from build123d import *

# Parameters (mm, degrees)
F0_R     = 13.5
F0_R_2   = 2.4852724595
F1_DEPTH = 7


with BuildPart() as f1:
    # F0 (on Top) → F1 (new body)
    with BuildSketch(Plane.XY):
        Circle(F0_R)
        with BuildLine():
            ThreePointArc((-11.0212433186, 4.5651484568), (-9.9188569362, 6.6275683173), (-8.4352944442, 8.4352944442))
            ThreePointArc((-8.4352944442, 8.4352944442), (-6.6275683173, 9.9188569362), (-4.5651484568, 11.0212433186))
            ThreePointArc((-4.5651484568, 11.0212433186), (-2.3272925012, 11.7000895011), (0, 11.9293078056))
            ThreePointArc((0, 11.9293078056), (2.3272925012, 11.7000895011), (4.5651484568, 11.0212433186))
            ThreePointArc((4.5651484568, 11.0212433186), (6.6275683173, 9.9188569362), (8.4352944442, 8.4352944442))
            ThreePointArc((8.4352944442, 8.4352944442), (9.9188569362, 6.6275683173), (11.0212433186, 4.5651484568))
            ThreePointArc((11.0212433186, 4.5651484568), (11.7000895011, 2.3272925012), (11.9293078056, 0))
            ThreePointArc((11.9293078056, 0), (11.7000895011, -2.3272925012), (11.0212433186, -4.5651484568))
            ThreePointArc((11.0212433186, -4.5651484568), (9.9188569362, -6.6275683173), (8.4352944442, -8.4352944442))
            ThreePointArc((8.4352944442, -8.4352944442), (6.6275683173, -9.9188569362), (4.5651484568, -11.0212433186))
            ThreePointArc((4.5651484568, -11.0212433186), (2.3272925012, -11.7000895011), (0, -11.9293078056))
            ThreePointArc((0, -11.9293078056), (-2.3272925012, -11.7000895011), (-4.5651484568, -11.0212433186))
            ThreePointArc((-4.5651484568, -11.0212433186), (-6.6275683173, -9.9188569362), (-8.4352944442, -8.4352944442))
            ThreePointArc((-8.4352944442, -8.4352944442), (-9.9188569362, -6.6275683173), (-11.0212433186, -4.5651484568))
            ThreePointArc((-11.0212433186, -4.5651484568), (-11.7000895011, -2.3272925012), (-11.9293078056, 0))
            ThreePointArc((-11.9293078056, 0), (-11.7000895011, 2.3272925012), (-11.0212433186, 4.5651484568))
        make_face(mode=Mode.SUBTRACT)
        with BuildLine():
            add(Edge.make_bspline(
                [(11.0212433186, 4.5651484568), (10.7307703614, 1.5514252721), (10.1663660438, -4.1433714543), (2.2942810987, -7.8104935299), (-0.1989491839, -4.6915291397), (-1.3315016332, -3.2145293013)],
                knots=[0, 0, 0, 0, 0.3754408897, 0.7085801344, 1, 1, 1, 1], degree=3))
            ThreePointArc((-1.3315016332, -3.2145293013), (-1.9330407592, -2.8929999397), (-2.4602942129, -2.4602942129))
            add(Edge.make_bspline(
                [(11.9293078056, 0), (10.5030009531, -2.6730846833), (7.8115947966, -7.7171301221), (-0.8744432081, -8.0954908894), (-1.9556350248, -4.2535609012), (-2.4602942129, -2.4602942129)],
                knots=[0, 0, 0, 0, 0.3754632807, 0.7084900303, 1, 1, 1, 1], degree=3))
            ThreePointArc((11.9293078056, 0), (11.7000895011, 2.3272925012), (11.0212433186, 4.5651484568))
        make_face()
        with BuildLine():
            add(Edge.make_bspline(
                [(4.5651484568, 11.0212433186), (6.4882912926, 8.6805285734), (10.1197801342, 4.2634610727), (7.1432551055, -3.9049968446), (3.1838363189, -3.436219375), (1.3315016332, -3.2145293013)],
                knots=[0, 0, 0, 0, 0.3754632807, 0.7084900303, 1, 1, 1, 1], degree=3))
            ThreePointArc((1.3315016332, -3.2145293013), (0.6787936462, -3.4125261045), (0, -3.4793814433))
            add(Edge.make_bspline(
                [(8.4352944442, 8.4352944442), (9.3162939954, 5.5368010983), (10.9810136566, 0.0662522262), (5.1051295916, -6.3413520413), (1.6264969852, -4.3930541604), (0, -3.4793814433)],
                knots=[0, 0, 0, 0, 0.3754632807, 0.7084900303, 1, 1, 1, 1], degree=3))
            ThreePointArc((8.4352944442, 8.4352944442), (6.6275683173, 9.9188569362), (4.5651484568, 11.0212433186))
        make_face()
        with BuildLine():
            add(Edge.make_bspline(
                [(-4.5651484568, 11.0212433186), (-1.5653669998, 10.7472190798), (4.1505997502, 10.2265263001), (7.9846135159, 1.9883168119), (4.7170514854, -0.2873495043), (3.2145293013, -1.3315016332)],
                knots=[0, 0, 0, 0, 0.3743391134, 0.7130961412, 1, 1, 1, 1], degree=3))
            ThreePointArc((3.2145293013, -1.3315016332), (2.8692477592, -1.968124113), (2.399653463, -2.5194758355))
            add(Edge.make_bspline(
                [(0, 11.9293078056), (2.6660813096, 10.5051188653), (7.7130575447, 7.806165889), (8.1160713079, -0.8810343308), (4.1864871277, -1.9887456195), (2.399653463, -2.5194758355)],
                knots=[0, 0, 0, 0, 0.3745960123, 0.7068535161, 1, 1, 1, 1], degree=3))
            ThreePointArc((0, 11.9293078056), (-2.3272925012, 11.7000895011), (-4.5651484568, 11.0212433186))
        make_face()
        with BuildLine():
            ThreePointArc((3.2145293013, 1.3315016332), (3.4125261045, 0.6787936462), (3.4793814433, 0))
            add(Edge.make_bspline(
                [(-8.4352944442, 8.4352944442), (-5.5290587898, 9.3115098739), (-0.061134709, 10.963342265), (6.2453098168, 5.1735666291), (4.3680084471, 1.6563982723), (3.4793814433, 0)],
                knots=[0, 0, 0, 0, 0.3758594316, 0.7069067859, 1, 1, 1, 1], degree=3))
            ThreePointArc((-8.4352944442, 8.4352944442), (-9.9188569362, 6.6275683173), (-11.0212433186, 4.5651484568))
            add(Edge.make_bspline(
                [(-11.0212433186, 4.5651484568), (-8.6805285734, 6.4882912926), (-4.2634610727, 10.1197801342), (3.9049968446, 7.1432551055), (3.436219375, 3.1838363189), (3.2145293013, 1.3315016332)],
                knots=[0, 0, 0, 0, 0.3754632807, 0.7084900303, 1, 1, 1, 1], degree=3))
        make_face()
        with BuildLine():
            ThreePointArc((1.3315016332, 3.2145293013), (1.9330407592, 2.8929999397), (2.4602942129, 2.4602942129))
            add(Edge.make_bspline(
                [(-11.9293078056, 0), (-10.5030009531, 2.6730846833), (-7.8115947966, 7.7171301221), (0.8744432081, 8.0954908894), (1.9556350248, 4.2535609012), (2.4602942129, 2.4602942129)],
                knots=[0, 0, 0, 0, 0.3754632807, 0.7084900303, 1, 1, 1, 1], degree=3))
            ThreePointArc((-11.9293078056, 0), (-11.7000895011, -2.3272925012), (-11.0212433186, -4.5651484568))
            add(Edge.make_bspline(
                [(-11.0212433186, -4.5651484568), (-10.7264528322, -1.5497162273), (-10.170190392, 4.1403306606), (-2.2901300579, 7.8138932667), (0.179003887, 4.6781669807), (1.3315016332, 3.2145293013)],
                knots=[0, 0, 0, 0, 0.3754632807, 0.7084900303, 1, 1, 1, 1], degree=3))
        make_face()
        with BuildLine():
            ThreePointArc((-1.3315016332, 3.2145293013), (-0.6787936462, 3.4125261045), (0, 3.4793814433))
            add(Edge.make_bspline(
                [(-8.4352944442, -8.4352944442), (-9.316899503, -5.5365868906), (-10.9804666932, -0.0667966119), (-5.1060517827, 6.3427012272), (-1.6248789699, 4.390564545), (0, 3.4793814433)],
                knots=[0, 0, 0, 0, 0.3754632807, 0.7084900303, 1, 1, 1, 1], degree=3))
            ThreePointArc((-8.4352944442, -8.4352944442), (-6.6275683173, -9.9188569362), (-4.5651484568, -11.0212433186))
            add(Edge.make_bspline(
                [(-4.5651484568, -11.0212433186), (-6.4889326824, -8.680562389), (-10.1190664786, -4.2637547057), (-7.1446234101, 3.9058904226), (-3.1813887332, 3.4345384579), (-1.3315016332, 3.2145293013)],
                knots=[0, 0, 0, 0, 0.3754632807, 0.7084900303, 1, 1, 1, 1], degree=3))
        make_face()
        with BuildLine():
            ThreePointArc((-3.2145293013, 1.3315016332), (-2.8929999397, 1.9330407592), (-2.4602942129, 2.4602942129))
            add(Edge.make_bspline(
                [(0, -11.9293078056), (-2.6939798135, -10.4868757597), (-7.7661281647, -7.7751649278), (-8.0802993691, 0.8709922033), (-4.2507900744, 1.9539046045), (-2.4602942129, 2.4602942129)],
                knots=[0, 0, 0, 0, 0.3765580427, 0.7085450955, 1, 1, 1, 1], degree=3))
            ThreePointArc((0, -11.9293078056), (2.3272925012, -11.7000895011), (4.5651484568, -11.0212433186))
            add(Edge.make_bspline(
                [(4.5651484568, -11.0212433186), (1.5497162273, -10.7264528322), (-4.1403306606, -10.170190392), (-7.8138932667, -2.2901300579), (-4.6781669807, 0.179003887), (-3.2145293013, 1.3315016332)],
                knots=[0, 0, 0, 0, 0.3754632807, 0.7084900303, 1, 1, 1, 1], degree=3))
        make_face()
        with BuildLine():
            add(Edge.make_bspline(
                [(11.0212433186, -4.5651484568), (8.680562389, -6.4889326824), (4.2637547057, -10.1190664786), (-3.9058904226, -7.1446234101), (-3.4345384579, -3.1813887332), (-3.2145293013, -1.3315016332)],
                knots=[0, 0, 0, 0, 0.3754632807, 0.7084900303, 1, 1, 1, 1], degree=3))
            ThreePointArc((-3.2145293013, -1.3315016332), (-3.4125261045, -0.6787936462), (-3.4793814433, 0))
            add(Edge.make_bspline(
                [(8.4352944442, -8.4352944442), (5.5284668219, -9.3179401167), (0.0480432269, -10.9832806768), (-6.3386089617, -5.1034639943), (-4.3895776289, -1.6246506872), (-3.4793814433, 0)],
                knots=[0, 0, 0, 0, 0.3758036016, 0.7085073702, 1, 1, 1, 1], degree=3))
            ThreePointArc((8.4352944442, -8.4352944442), (9.9188569362, -6.6275683173), (11.0212433186, -4.5651484568))
        make_face()
        with BuildLine():
            ThreePointArc((3.2145293013, -1.3315016332), (3.4125261045, -0.6787936462), (3.4793814433, 0))
            ThreePointArc((3.4793814433, 0), (3.4125261045, 0.6787936462), (3.2145293013, 1.3315016332))
            ThreePointArc((3.2145293013, 1.3315016332), (2.8929999397, 1.9330407592), (2.4602942129, 2.4602942129))
            ThreePointArc((2.4602942129, 2.4602942129), (1.9330407592, 2.8929999397), (1.3315016332, 3.2145293013))
            ThreePointArc((1.3315016332, 3.2145293013), (0.6787936462, 3.4125261045), (0, 3.4793814433))
            ThreePointArc((0, 3.4793814433), (-0.6787936462, 3.4125261045), (-1.3315016332, 3.2145293013))
            ThreePointArc((-1.3315016332, 3.2145293013), (-1.9330407592, 2.8929999397), (-2.4602942129, 2.4602942129))
            ThreePointArc((-2.4602942129, 2.4602942129), (-2.8929999397, 1.9330407592), (-3.2145293013, 1.3315016332))
            ThreePointArc((-3.2145293013, 1.3315016332), (-3.4125261045, 0.6787936462), (-3.4793814433, 0))
            ThreePointArc((-3.4793814433, 0), (-3.4125261045, -0.6787936462), (-3.2145293013, -1.3315016332))
            ThreePointArc((-3.2145293013, -1.3315016332), (-2.8929999397, -1.9330407592), (-2.4602942129, -2.4602942129))
            ThreePointArc((-2.4602942129, -2.4602942129), (-1.9330407592, -2.8929999397), (-1.3315016332, -3.2145293013))
            ThreePointArc((-1.3315016332, -3.2145293013), (-0.6787936462, -3.4125261045), (0, -3.4793814433))
            ThreePointArc((0, -3.4793814433), (0.6787936462, -3.4125261045), (1.3315016332, -3.2145293013))
            ThreePointArc((1.3315016332, -3.2145293013), (1.8976707876, -2.9163231662), (2.399653463, -2.5194758355))
            ThreePointArc((2.399653463, -2.5194758355), (2.8692477592, -1.968124113), (3.2145293013, -1.3315016332))
        make_face()
        Circle(F0_R_2, mode=Mode.SUBTRACT)
    extrude(amount=F1_DEPTH)


solid = f1.part
Design review of the part built by this model. Coordinates are the model's own, in mm. Round coordinates to 2 decimals unless told otherwise and drop trailing zeros. Answer as a JSON object with one key per item and string values.
Item 1: We need section A-A on y = -0.5. State how many separate pieces and enclosed holes the cut face has, and give its area (3 significant figures).
Answer sheet:
{"separate pieces": "9", "enclosed holes": "0", "area": "104 mm^2"}
Item 2: Clearance check with a flat-ended pin moving along its axis: P1, Ø1, axis at x = 7, z = 6.5, coming from the -Y side. State where the tip first meets the part, or that it passes through.
Answer sheet:
{"P1": "stops at y = -11.83"}
Item 3: The part is to be moulded in two halves that separate along X. For faces 1 (the cylindrical face through (-3.41, 0.69, 3.45)), 2 (the flat face through (0, -3, 7)), 3 (the cylindrical face through (-2.93, -13.18, 3.45)), say which applies: pulls with the +X half, pulls with the -X half, needs draft (parallel to the pull), parting line crosses it, or undercut.
Answer sheet:
{"face 1": "undercut", "face 2": "needs draft", "face 3": "parting line crosses it"}
